CAD build for the part. Positions are in the model's coordinates, mm. A direction names the side the tool comes from. Round coordinates to 2 decimals unless told otherwise and drop trailing zeros. Loops run counter-clockwise (first coordinate to the right, second up) from the corner with the lowest first, then second, coordinate; pieces in that order, holes last.
from build123d import *

# Parameters (mm, degrees)
F1_DEPTH = 40


with BuildPart() as f1:
    # F0 (on Top) → F1 (new body)
    with BuildSketch(Plane.XY):
        with BuildLine():
            Line((66, 0), (6, 0))
            ThreePointArc((6, 0), (1.757359, -1.757359), (0, -6))
            Line((0, -6), (0, -42.973471))
            ThreePointArc((0, -42.973471), (1.813257, -47.271283), (6.157062, -48.971415))
            Line((6.157062, -48.971415), (62.133626, -47.505617))
            ThreePointArc((62.133626, -47.505617), (64.277221, -48.328466), (65.211129, -50.426058))
            Line((65.211129, -50.426058), (65.813199, -73.418177))
            ThreePointArc((65.813199, -73.418177), (64.99035, -75.561771), (62.892758, -76.49568))
            Line((62.892758, -76.49568), (57.894471, -76.626564))
            Line((57.894471, -76.626564), (57.81594, -73.627593))
            Line((57.81594, -73.627593), (61.814569, -73.522885))
            ThreePointArc((61.814569, -73.522885), (61.191964, -72.12449), (59.762901, -71.575924))
            Line((59.762901, -71.575924), (57.763586, -71.628278))
            ThreePointArc((57.763586, -71.628278), (56.365191, -72.250883), (55.816626, -73.679946))
            Line((55.816626, -73.679946), (55.895156, -76.678918))
            Line((55.895156, -76.678918), (2.913318, -78.066297))
            Line((2.913318, -78.066297), (2.80861, -74.067667))
            Line((2.80861, -74.067667), (1.808953, -74.093844))
            ThreePointArc((1.808953, -74.093844), (0.410558, -74.71645), (-0.138008, -76.145513))
            Line((-0.138008, -76.145513), (-0.059477, -79.144485))
            ThreePointArc((-0.059477, -79.144485), (1.185734, -81.941274), (4.04386, -83.038406))
            Line((4.04386, -83.038406), (65.022957, -81.441612))
            ThreePointArc((65.022957, -81.441612), (69.218142, -79.573796), (70.863839, -75.286607))
            Line((70.863839, -75.286607), (70.157062, -48.295859))
            ThreePointArc((70.157062, -48.295859), (68.289245, -44.100675), (64.002056, -42.454977))
            Line((64.002056, -42.454977), (8.078531, -43.919386))
            ThreePointArc((8.078531, -43.919386), (5.906629, -43.06932), (5, -40.920414))
            Line((5, -40.920414), (5, -8))
            ThreePointArc((5, -8), (5.87868, -5.87868), (8, -5))
            Line((8, -5), (70, -5))
            Line((70, -5), (70, -4))
            ThreePointArc((70, -4), (68.828427, -1.171573), (66, 0))
        make_face()
    extrude(amount=F1_DEPTH)


solid = f1.part
Item 1: 3-axis set-ups, long thin cutter, end or side, ignore diameter. For faces 1 (the cylindrical face through (65.01, -75.54, 19.72)), 2 (the cylindrical face through (5.86, -5.9, 19.72)), 3 (the cylindrical face through (56.38, -72.235, 19.72)): which of +Z, -Z, +X, -X, +Y, -Y reach the whole face in a straight line?
Verdict:
face 1: +Z, -Z
face 2: +Z, -Z, +X
face 3: +Z, -Z, -X
Item 2: Cut at C-C (y = -22). List the corners of the cut face in (x, z).
Verdict:
outline: (0, 0) - (5, 0) - (5, 40) - (0, 40) - close
Item 3: Wall check: L1, parallel to Y at x = 32.5, z = 33.5; L2, parallel to Y at x = 12, z = 11; L3, parallel to X at y = -14, z = 30.5. Give the ranges that are in metal, low to high.
Verdict:
L1: y = -82.29 to -77.29, -48.28 to -43.28, -5 to 0
L2: y = -82.83 to -77.83, -48.82 to -43.82, -5 to 0
L3: x = 0 to 5
Item 4: Cut at A-A (x = 15.5). List the corners of the cut face in (y, z), plus the area to 3 significant figures.
Verdict:
outline: (-82.74, 0) - (-77.74, 0) - (-77.74, 40) - (-82.74, 40) - close; (-48.73, 0) - (-43.73, 0) - (-43.73, 40) - (-48.73, 40) - close; (-5, 0) - (0, 0) - (0, 40) - (-5, 40) - close
area: 600 mm2
Item 5: Cut at D-D (y = -66). List the corners of the cut face in (x, z), plus the area to 3 significant figures.
Verdict:
outline: (65.62, 0) - (70.62, 0) - (70.62, 40) - (65.62, 40) - close
area: 200 mm2
Item 6: Flat gauge pins, fed straight in: P1, Ø1.1, axis at y = -4.5, z = 22, coming from the +X side; P2, Ø3, axis at x = 42, z = 29, coming from the -Y side; P3, Ø11, axis at y = -30.5, z = 29, coming from the -X side. Where does each tip first touch, or does it go through?
Verdict:
P1: stops at x = 70
P2: stops at y = -82.08
P3: stops at x = 0
Item 7: Mould opens along Y. For faces 4 (the cylindrical face through (61.21, -72.14, 19.72)), 5 (the flat face through (0, -24, 20)), 6 (the flat face through (36, 0, 20)) say: released by +Y, released by -Y, zero draft, split by the parting line, or undercut.
Verdict:
face 4: undercut
face 5: zero draft
face 6: released by +Y
